```python
from build123d import *

# Parameters (mm, degrees)
BOSS_EXTRUDE1_DEPTH = 12
SKETCH2_R           = 2
CUT_EXTRUDE4_DEPTH  = 12
CUT_EXTRUDE5_START  = -77
SKETCH2_3_R         = 2
CUT_EXTRUDE5_DEPTH  = 12


with BuildPart() as part:
    # Sketch1 → Boss-Extrude1 (new body)
    with BuildSketch(Plane(origin=(0, 0, 0), x_dir=(1, 0, 0), z_dir=(0, 1, 0))):
        with BuildLine():
            ThreePointArc((-30.343379621, 16.417347933), (0, 34.5), (30.343379621, 16.417347933))
            Line((30.343379621, 16.417347933), (25.624396188, 44.057108045))
            ThreePointArc((25.624396188, 44.057108045), (24.064523617, 40.171296717), (19.893289621, 39.805866754))
            ThreePointArc((19.893289621, 39.805866754), (0, 44.5), (-19.893289621, 39.805866754))
            ThreePointArc((-19.893289621, 39.805866754), (-24.064523617, 40.171296717), (-25.624396188, 44.057108045))
            Line((-25.624396188, 44.057108045), (-30.343379621, 16.417347933))
        make_face()
        Polygon((20, 77), (25.624396188, 44.057108045), (34, -5), (49, -5), (49, 0), (39, 0), (25, 82), (-25, 82), (-39, 0), (-49, 0), (-49, -5), (-34, -5), (-25.624396188, 44.057108045), (-20, 77), align=None)
    extrude(amount=BOSS_EXTRUDE1_DEPTH)

    # Sketch2 → Cut-Extrude4 (cut)
    with BuildSketch(Plane.XY):
        with Locations((44, 6)):
            Circle(SKETCH2_R)
        with Locations((-44, 6)):
            Circle(SKETCH2_R)
    extrude(amount=CUT_EXTRUDE4_DEPTH, mode=Mode.SUBTRACT)

    # Sketch2_3 → Cut-Extrude5 (cut)
    with BuildSketch(Plane.XY.offset(CUT_EXTRUDE5_START)):
        with Locations((-20, 6)):
            Circle(SKETCH2_3_R)
        with Locations((20, 6)):
            Circle(SKETCH2_3_R)
    extrude(amount=-CUT_EXTRUDE5_DEPTH, mode=Mode.SUBTRACT)


solid = part.part
```
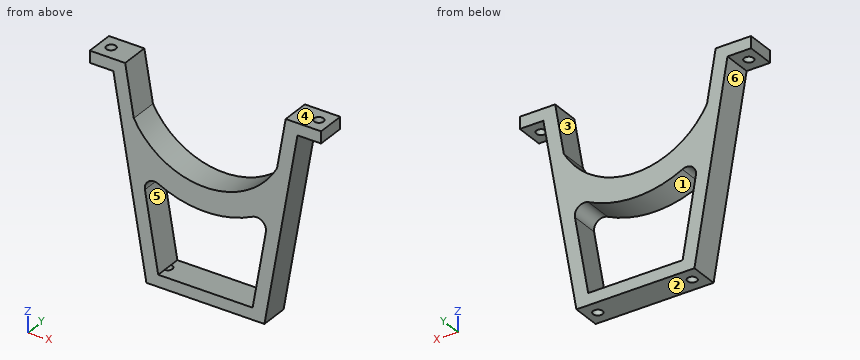
Design review of the part built by this model. Coordinates are the model's own, in mm. Face numbers are marked on the shaded views. A direction names the side the tool comes from. Coordinates: 2 decimals unless noted, no trailing zeros. Order: outer loops, then holes, each group sorted by start corner. A loop starts at its lowest first (then second) coordinate and runs counter-clockwise, first axis right, second up. Notation, with made-up numbers: (-36.75, -33.75) - (16.25, -33.75) arc R7 ccw to (16.25, -21.75) - close; hole circle Ø5 at (63.25, 7.5). An arc over 180 degrees is marked (long way). One line per question, with ' | ' between items.
Q1. Consider section A-A, the plane x = -44. Give the boundary of the cut face in (y, z), then the cut area to 3 significant figures.
Answer key:
outline: (0, 0) - (4, 0) - (4, 5) - (0, 5) - close; (8, 0) - (12, 0) - (12, 5) - (8, 5) - close | area: 40.0 mm2
Q2. Consider section C-C, the plane z = -70.5. Give the boundary of the cut face in (x, y), then the cut area to 3 significant figures.
Answer key:
outline: (-26.96, 0) - (-21.11, 0) - (-21.11, 12) - (-26.96, 12) - close; (21.11, 0) - (26.96, 0) - (26.96, 12) - (21.11, 12) - close | area: 140 mm2
Q3. To check wall thickness, follow line 1 along X through (y, z) = (6, -78.5); line 2 along Y through (x, z) = (-44, 3.3); line 3 along X through (y, z) = (6, -77.95). State the ranges of each line that lie inside material, in increasing order.
Answer key:
line 1: x = -25.6 to -22, -18 to 18, 22 to 25.6 | line 2: y = 0 to 4, 8 to 12 | line 3: x = -25.69 to -22, -18 to 18, 22 to 25.69
Q4. Consider section B-B, the plane z = -42. Give the boundary of the cut face in (x, y), then the cut area to 3 significant figures.
Answer key:
outline: (-31.83, 0) - (-25.43, 0) - (-25.43, 12) - (-31.83, 12) - close; (-14.71, 0) - (14.71, 0) - (14.71, 12) - (-14.71, 12) - close; (25.43, 0) - (31.83, 0) - (31.83, 12) - (25.43, 12) - close | area: 506 mm2
Q5. The part is to be moulded in two halves that separate along X. For the marked faces 4, 5 and 6, say which applies: +X half, -X half, draft (parallel to the pull), parting line (faces both ways), or undercut.
Answer key:
face 4: draft | face 5: undercut | face 6: -X half
Q6. For the marked faces 1, 2 and 3, list the 3-axis set-ups (+Z, -Z, +X, -X, +Y, -Y) from which the entire face can be reached by the end or side of a thin tool; tool diameter is ignored.
Answer key:
face 1: +Y, -Y | face 2: -Z, +X, -X, +Y, -Y | face 3: +Z, +Y, -Y
Q7. Clearance check with flat-ended pins moving along their axes: pin 1 Ø0.6 at (x, y) = (21.5, 5.5) entering from -Z; pin 2 Ø3 at (y, z) = (6.5, -52) entering from -X; pin 3 Ø6 at (x, y) = (9, 1.5) entering from +Z; pin 4 Ø6.5 at (x, y) = (44, 6) entering from +Z. State where each tip first meets the part, or that it passes through.
Answer key:
pin 1: stops at z = -77 | pin 2: stops at x = -30.38 | pin 3: stops at z = -32.35 | pin 4: stops at z = 5
